The drawing under review shows one solid part. Ordinate dimensions are in mm from its lowest x, y, z. A direction names the side the tool comes from. Coordinates: 2 decimals unless noted, no trailing zeros. Loops run counter-clockwise (first coordinate to the right, second up) from the corner with the lowest first, then second, coordinate; pieces in that order, holes last. Notation, with made-up numbers: M 27,76.5 L 72,76.5 A25 cw 72,95.5 Z; hole C 89.5,64.25 d4. An arc over 180 degrees is marked long. Put each result on its own line as item: value.
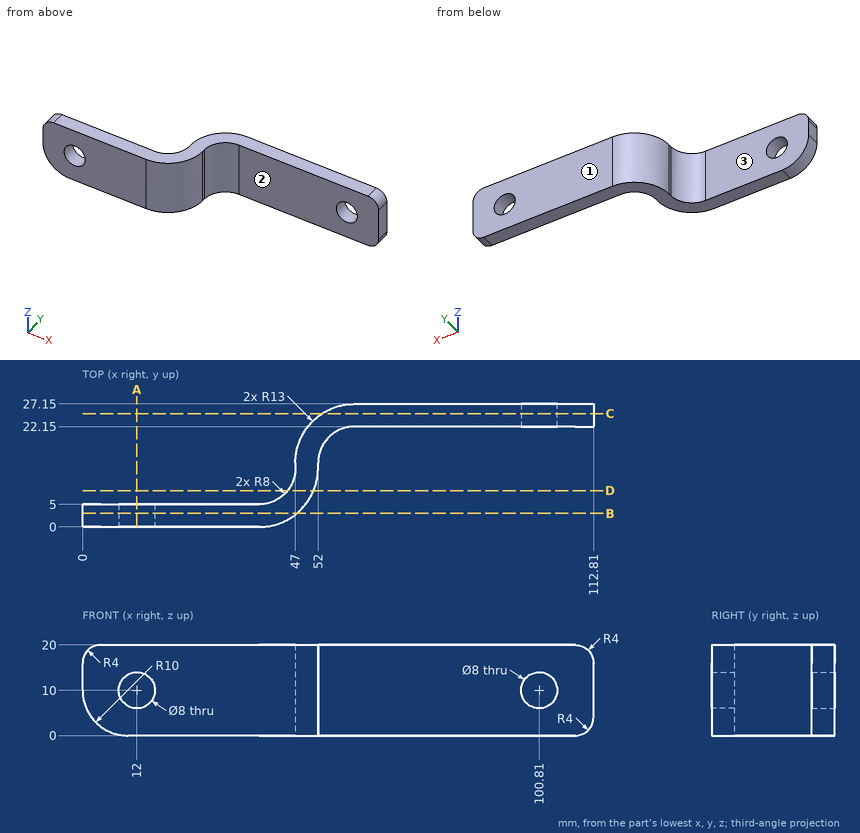
(1) Wall thickness on line 1 along Z through (x, y) = (100.81, 24.95); line 2 along Y through (x, z) = (8, 2.25); line 3 along X through (y, z) = (1.35, 10): over which ranges is each line inside the solid? List them lowest first. Write a range as [from, to].
Determined:
line 1: z = [0, 6], [14, 20]
line 2: y = [0, 5]
line 3: x = [0, 8], [16, 44.77]
(2) Tool access review of the marked faces 1, 2 and 3: name each direction out of +Z, -Z, +X, -X, +Y, -Y from which nothing blocks a thin tool from reaching the whole face with its end or side.
Determined:
face 1: +Z, -Z, +X, -X, +Y
face 2: +Z, -Z, +X, -Y
face 3: +Z, -Z, -X, +Y
(3) Add section C-C (y = 25). Write out the cut boundary in (x, z).
Determined:
outline: M 52.84,0 L 108.81,0 A4 ccw 112.81,4 L 112.81,16 A4 ccw 108.81,20 L 52.84,20 Z; hole C 100.81,10 d8
(4) Add section B-B (y = 3). Write out the cut boundary in (x, z), plus the area to 3 significant figures.
Determined:
outline: M 0,10 A10 ccw 10,0 L 47.31,0 L 47.31,20 L 4,20 A4 ccw 0,16 Z; hole C 12,10 d8
area: 871 mm^2
(5) Add section D-D (y = 8). Write out the cut boundary in (x, z) (3 decimals), plus the area to 3 significant figures.
Determined:
outline: M 45.245,0 L 51,0 L 51,20 L 45.245,20 Z
area: 115 mm^2
(6) Add section A-A (x = 12). Write out the cut boundary in (y, z).
Determined:
outline: M 0,0 L 5,0 L 5,6 L 0,6 Z; M 0,14 L 5,14 L 5,20 L 0,20 Z
(7) For pin 1 (3 mm diameter, centred on y = 7.5, z = 15.5, fed in from -X); pin 2 (1 mm diameter, centred on x = 91.5, z = 11.5, fed in from -Y); pin 3 (10 mm diameter, centred on y = 13.5, z = 17, fed in from +X), all flat-tipped, find the tip position at first contact; note any pin that passes through.
Determined:
pin 1: stops at x = 42.87
pin 2: stops at y = 22.15
pin 3: stops at x = 53.29
